Answer from the drawing. Dimensions are ordinates in mm from the lowest x, y and z of the part. Give positions to 0.01 mm unless a question says otherwise; leave off trailing zeros. Loops run counter-clockwise (first coordinate to the right, second up) from the corner with the lowest first, then second, coordinate; pieces in that order, holes last.
(1) Find section B-B, the plane x = 21. Write down the section's boundary in (y, z).
(2) Find section D-D, the plane z = 13.5. Write down the section's boundary in (x, y), then the cut area to 3 significant figures.
(3) Straight lines are drawn through the part: probe 1 along Y at (x, z) = (30.5, 12.5); probe 2 along Y at (x, z) = (4.5, 14); probe 3 along Y at (x, z) = (38, 1.75). For each, find the intervals that lie inside material, in ascending order.
(4) Each of these flat-tipped pins is pushed along its axis until it touches: P1, Ø8, axis at y = 17.5, z = 13, coming from the -X side; P2, Ø1, axis at x = 40.5, y = 19, coming from the -Z side; P3, Ø1, axis at x = 35.5, y = 14, coming from the -Z side; P4, Ø1, axis at x = 7.5, y = 15, coming from the -Z side. Where does it stop, or does it pass through?
(5) Find section C-C, the plane z = 19.5. Write down the section's boundary in (x, y).
(6) Find section A-A, the plane y = 12.5. Write down the section's boundary in (x, z), then the cut area to 3 significant figures.
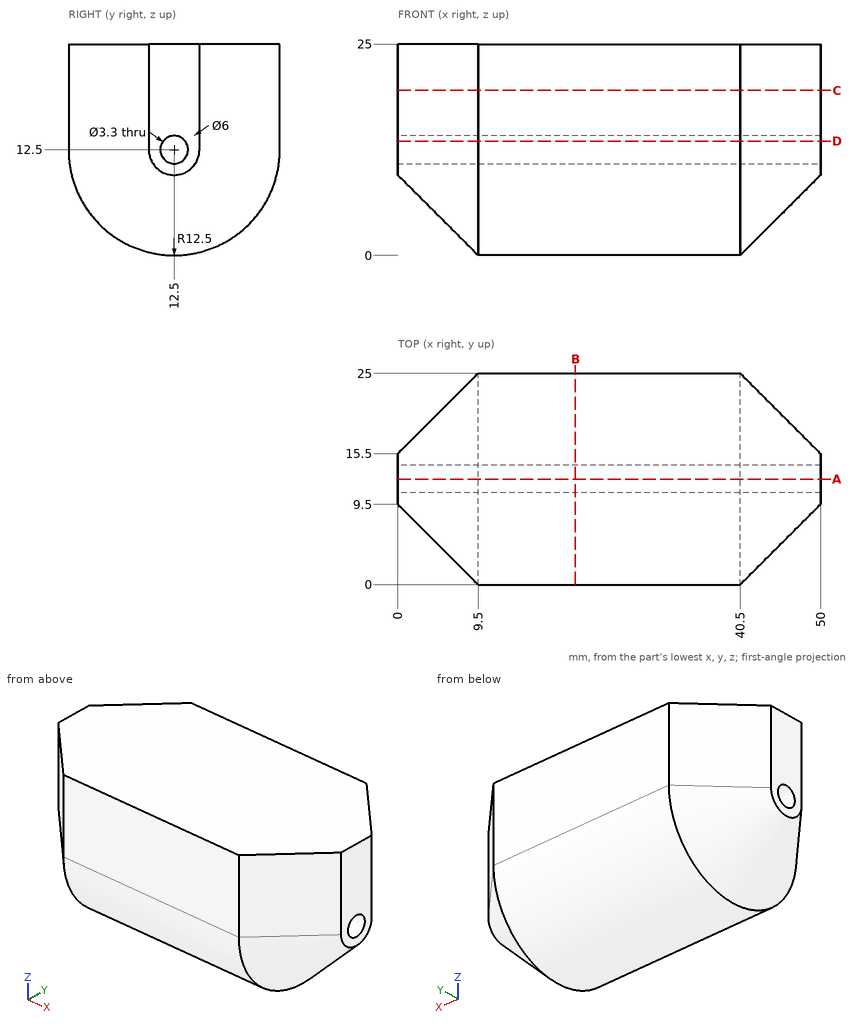
Entries:
1. outline: (0, 12.5) arc R12.5 ccw to (25, 12.5) - (25, 25) - (0, 25) - close; hole circle Ø3.3 at (12.5, 12.5)
2. outline: (0, 9.5) - (9.5, 0) - (40.5, 0) - (50, 9.5) - (50, 11.19) - (0, 11.19) - close; (0, 13.81) - (50, 13.81) - (50, 15.5) - (40.5, 25) - (9.5, 25) - (0, 15.5) - close
2. area: 938 mm2
3. probe 1: y = 0 to 10.85, 14.15 to 25
3. probe 2: y = 5 to 11.81, 13.19 to 20
3. probe 3: y = 6.12 to 18.88
4. P1: stops at x = 0
4. P2: stops at z = 1.53
4. P3: stops at z = 0.04
4. P4: stops at z = 1.78
5. outline: (0, 9.5) - (9.5, 0) - (40.5, 0) - (50, 9.5) - (50, 15.5) - (40.5, 25) - (9.5, 25) - (0, 15.5) - close
6. outline: (0, 9.5) - (9.5, 0) - (40.5, 0) - (50, 9.5) - (50, 10.85) - (0, 10.85) - close; (0, 14.15) - (50, 14.15) - (50, 25) - (0, 25) - close
6. area: 995 mm2
